```python
from build123d import *

# Parameters (mm, degrees)
CROQUIS1_R              = 1.5
SALIENTE_EXTRUIR1_DEPTH = 2


with BuildPart() as part:
    # Croquis1 → Saliente-Extruir1 (new body)
    # profile 1 of 3: a face of its own
    with BuildSketch(Plane(origin=(0, 0, 0), x_dir=(1, 0, 0), z_dir=(0, 1, 0))):
        Polygon((-29, -16), (-29, 0), (-29, 16), (0, 16), (29, 16), (29, 0), (29, -16), (0, -16), align=None)
    # profile 2 of 3: a face of its own
    with BuildSketch(Plane(origin=(0, 0, 0), x_dir=(1, 0, 0), z_dir=(0, 1, 0))):
        with BuildLine():
            Line((31, 3.5), (29, 3.5))
            Line((29, 3.5), (29, 0))
            Line((29, 0), (29, -3.5))
            Line((29, -3.5), (31, -3.5))
            ThreePointArc((31, -3.5), (34.5, 0), (31, 3.5))
        make_face()
        with Locations(Location((31, 0, 0), (0, 0, 270))):
            Circle(CROQUIS1_R, mode=Mode.SUBTRACT)
    # profile 3 of 3: a face of its own
    with BuildSketch(Plane(origin=(0, 0, 0), x_dir=(1, 0, 0), z_dir=(0, 1, 0))):
        with BuildLine():
            Line((-29, -3.5), (-29, 0))
            Line((-29, 0), (-29, 3.5))
            Line((-29, 3.5), (-31, 3.5))
            ThreePointArc((-31, 3.5), (-34.5, 0), (-31, -3.5))
            Line((-31, -3.5), (-29, -3.5))
        make_face()
        with Locations(Location((-31, 0, 0), (0, 0, 270))):
            Circle(CROQUIS1_R, mode=Mode.SUBTRACT)
    extrude(amount=SALIENTE_EXTRUIR1_DEPTH)


solid = part.part
```
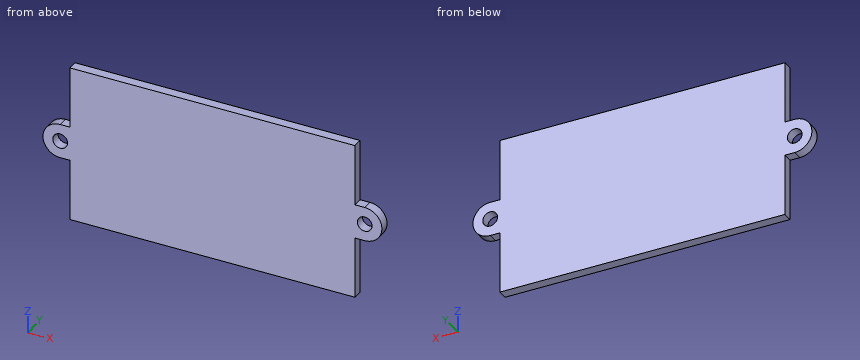
Could you check a few things on this model? Use its own coordinates, in mm. Coordinates: 2 decimals unless noted, no trailing zeros. Write each loop counter-clockwise with the first axis right and the second up, starting at its lowest first coordinate (ties: lowest second). Pieces come first, ordered by that corner, then holes. Notation, with made-up numbers: (17, 49.25) -> (26, 49.25) arc R23 ccw to (26, 83.25) -> close; hole circle Ø8 at (61, 52). An arc over 180 degrees is marked (long way). One line per question, with ' | ' between items. Start each with the question number.
1. If we section it at B-B (y = 0.9): Please give me the cut outline in (x, z).
2. If we section it at C-C (z = 8): Please give me the cut outline in (x, y).
3. Please list where these lines run through material, in increasing order: line 1 along X through (y, z) = (0.6, 0); line 2 along X through (y, z) = (1.35, 1); line 3 along X through (y, z) = (1.5, -9.5).
4. Will these pins go through, and if not, where does the flat tip stop? P1, Ø1.8, axis at x = 31, z = 0, coming from the -Y side; P2, Ø1, axis at y = 1.5, z = -2, coming from the -X side; P3, Ø0.6, axis at y = 1, z = -8.5, coming from the +X side; P4, Ø0.6, axis at x = -30, y = 1, coming from the -Z side.
5. If we section it at A-A (z = 0): Please give me the cut outline in (x, y), and give its area (3 significant figures).
Return value:
1) outline: (-31, -3.5) -> (-29, -3.5) -> (-29, -16) -> (29, -16) -> (29, -3.5) -> (31, -3.5) arc R3.5 ccw to (31, 3.5) -> (29, 3.5) -> (29, 16) -> (-29, 16) -> (-29, 3.5) -> (-31, 3.5) arc R3.5 ccw to start; hole circle Ø3 at (-31, 0); hole circle Ø3 at (31, 0)
2) outline: (-29, 0) -> (29, 0) -> (29, 2) -> (-29, 2) -> close
3) line 1: x = -34.5 to -32.5, -29.5 to 29.5, 32.5 to 34.5 | line 2: x = -34.35 to -32.12, -29.88 to 29.88, 32.12 to 34.35 | line 3: x = -29 to 29
4) P1: passes through | P2: stops at x = -34.16 | P3: stops at x = 29 | P4: stops at z = -3.5
5) outline: (-34.5, 0) -> (-32.5, 0) -> (-32.5, 2) -> (-34.5, 2) -> close; (-29.5, 0) -> (29.5, 0) -> (29.5, 2) -> (-29.5, 2) -> close; (32.5, 0) -> (34.5, 0) -> (34.5, 2) -> (32.5, 2) -> close | area: 126 mm²
